```python
from build123d import *

# Parameters (mm, degrees)
F0_W     = 50.8
F0_H     = 50.8
F1_DEPTH = 50.8
F2_R     = 12.7
F3_DEPTH = 50.8
F4_W     = 25.4
F4_H     = 25.4
F5_DEPTH = 12.7


with BuildPart() as f1:
    # F0 (on Right) → F1 (new body)
    with BuildSketch(Plane.YZ):
        with Locations((-33.802004, 33.420096)):
            Rectangle(F0_W, F0_H)
    extrude(amount=F1_DEPTH)

    # F2 (on face) → F3 (cut)
    with BuildSketch(Plane.YZ.offset(50.8)):
        with Locations((-34.011841, 35.279486)):
            Circle(F2_R)
    extrude(amount=-F3_DEPTH, mode=Mode.SUBTRACT)

    # F4 (on face) → F5 (join)
    with BuildSketch(Plane(origin=(0, -8.402004, 0), x_dir=(-1, 0, 0), z_dir=(0, 1, 0))):
        with Locations((-26.066826, 37.524144)):
            Rectangle(F4_W, F4_H)
    extrude(amount=F5_DEPTH)


solid = f1.part
```
The listing builds one solid part. Answer for the finished solid, in the listing's coordinates (mm). A direction names the side the tool comes from. Give positions to 0.01 mm unless a question says otherwise; leave off trailing zeros. Order: outer loops, then holes, each group sorted by start corner. A loop starts at its lowest first (then second) coordinate and runs counter-clockwise, first axis right, second up.
Item 1: The part is cut by section A-A, the plane z = 40. Give the vertices of the cut face in (x, y).
From the geometry:
outline: (0, -59.2) - (50.8, -59.2) - (50.8, -45.8) - (0, -45.8) - close; (0, -22.22) - (50.8, -22.22) - (50.8, -8.4) - (38.77, -8.4) - (38.77, 4.3) - (13.37, 4.3) - (13.37, -8.4) - (0, -8.4) - close
Item 2: Which of the six approach directions +Z, -Z, +X, -X, +Y, -Y give full straight-line access (tool end or side, diameter ignored) to faces 1 (the face through (25, -34, 58.82)), 2 (the face through (26, -2, 24.824)), 3 (the face through (0, -34, 22)), 4 (the face through (38.767, -2, 37)), 5 (the face through (26, -2, 50.224))?
From the geometry:
face 1: +Z, +X, -X, +Y, -Y
face 2: -Z, +X, -X, +Y
face 3: +Z, -Z, -X, +Y, -Y
face 4: +Z, -Z, +X, +Y
face 5: +Z, +X, -X, +Y
Item 3: The part is cut by section D-D, the plane z = 45.5. Give the vertices of the cut face in (x, y), and give its area (3 significant figures).
From the geometry:
outline: (0, -59.2) - (50.8, -59.2) - (50.8, -41.55) - (0, -41.55) - close; (0, -26.47) - (50.8, -26.47) - (50.8, -8.4) - (38.77, -8.4) - (38.77, 4.3) - (13.37, 4.3) - (13.37, -8.4) - (0, -8.4) - close
area: 2,140 mm2
Item 4: The part is cut by section B-B, the plane y = -35. Give the vertices of the cut face in (x, z), and give its area (3 significant figures).
From the geometry:
outline: (0, 8.02) - (50.8, 8.02) - (50.8, 22.62) - (0, 22.62) - close; (0, 47.94) - (50.8, 47.94) - (50.8, 58.82) - (0, 58.82) - close
area: 1,290 mm2
Item 5: The part is cut by section C-C, the plane x = 26. Give the vertices of the cut face in (y, z), and give its area (3 significant figures).
From the geometry:
outline: (-59.2, 8.02) - (-8.4, 8.02) - (-8.4, 24.82) - (4.3, 24.82) - (4.3, 50.22) - (-8.4, 50.22) - (-8.4, 58.82) - (-59.2, 58.82) - close; hole circle Ø25.4 at (-34.01, 35.28)
area: 2,400 mm2
Item 6: Given pin 1 Ø2 at (x, z) = (25, 15.5) entering from +Y; pin 2 Ø6.5 at (x, y) = (28, -1) entering from -Z; pin 3 Ø14 at (y, z) = (1, 34.5) entering from +X, each flat-ended and moving along its own axis, determine where each tip first touches the part or whether it passes through.
From the geometry:
pin 1: stops at y = -8.4
pin 2: stops at z = 24.82
pin 3: stops at x = 38.77
Item 7: For a pull along Z with two mould halves and no side action, classify faces 6 (the face through (13.367, -2, 37)), 7 (the face through (25.8, -27.2, 46)), 8 (the face through (25, -34, 8.02)) as pulls with the +Z half, pulls with the -Z half, needs draft (parallel to the pull), parting line crosses it, or undercut.
From the geometry:
face 6: needs draft
face 7: undercut
face 8: pulls with the -Z half
Item 8: Find the intervals of material crossed by probe 1 along Y at (x, z) = (6, 55); probe 2 along Y at (x, z) = (6, 41.5); probe 3 along Z at (x, y) = (33, -37.5), in increasing order.
From the geometry:
probe 1: y = -59.2 to -8.4
probe 2: y = -59.2 to -45.08, -22.94 to -8.4
probe 3: z = 8.02 to 23.07, 47.49 to 58.82
